For this review, take the finished solid that the model builds, in its own axes (mm). Face numbers are marked on the shaded views. Round coordinates to 2 decimals unless told otherwise and drop trailing zeros. Loops run counter-clockwise (first coordinate to the right, second up) from the corner with the lowest first, then second, coordinate; pieces in that order, holes last. Notation, with made-up numbers: (7, 24) -> (50, 24) arc R18 cw to (50, 31) -> close; hole circle Ø11 at (18, 74). An arc over 180 degrees is marked (long way). Write each question's results on one line, items separated by ' | '.
```python
from build123d import *

# Parameters (mm, degrees)
SKETCH1_W               = 88.9
SKETCH1_H               = 41.275
BOSS_EXTRUDE1_DEPTH     = 12.7
F_1_4_CLEARANCE_HOLE1_D = 6.7564
FILLET1_R               = 3.175


with BuildPart() as part:
    # Sketch1 → Boss-Extrude1 (new body)
    with BuildSketch(Plane(origin=(0, 0, 0), x_dir=(1, 0, 0), z_dir=(0, 1, 0))):
        with Locations((44.45, 20.6375)):
            Rectangle(SKETCH1_W, SKETCH1_H)
    extrude(amount=BOSS_EXTRUDE1_DEPTH)

    # 1/4 Clearance Hole1 (through all)
    with Locations(Plane(origin=(0, 12.7, 0), x_dir=(1, 0, 0), z_dir=(0, 1, 0))):
        with Locations((73.025, 31.75)):
            Hole(F_1_4_CLEARANCE_HOLE1_D / 2)

    # Fillet1
    fillet1_edges = [part.edges().sort_by_distance(p)[0] for p in [
        (0, 6.35, -41.275),
        (88.9, 6.35, -41.275),
        (88.9, 6.35, 0),
        (0, 6.35, 0),
    ]]
    fillet(fillet1_edges, radius=FILLET1_R)


solid = part.part
```
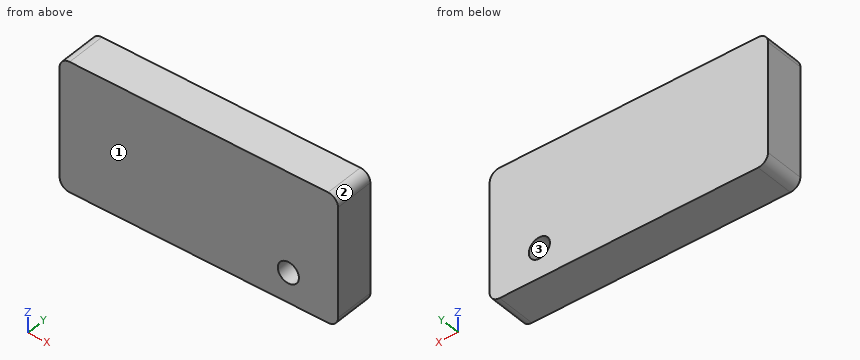
1. Draft analysis for pull direction Z (two halves, no side actions). For the marked faces 1, 2 and 3, state which applies: released by +Z, released by -Z, zero draft, split by the parting line, or undercut.
Values found:
face 1: zero draft | face 2: released by +Z | face 3: undercut
2. Consider section B-B (x = 71). State the section outline as (y, z) points (3 decimals).
Values found:
outline: (0, -41.275) -> (12.7, -41.275) -> (12.7, -34.454) -> (0, -34.454) -> close; (0, -29.046) -> (12.7, -29.046) -> (12.7, 0) -> (0, 0) -> close
3. To check wall thickness, follow probe 1 along X at (y, z) = (4, -31.75); probe 2 along Z at (x, y) = (72, 9.75) (3 decimals). State the ranges of each line that lie inside material, in increasing order.
Values found:
probe 1: x = 0 to 69.65, 76.4 to 88.9 | probe 2: z = -41.275 to -34.969, -28.531 to 0
4. Consider section A-A (z = -31.75). State the section outline as (x, y) points, plus the area to 3 significant figures.
Values found:
outline: (0, 0) -> (69.65, 0) -> (69.65, 12.7) -> (0, 12.7) -> close; (76.4, 0) -> (88.9, 0) -> (88.9, 12.7) -> (76.4, 12.7) -> close | area: 1,040 mm2
